Here's how the part is built. I have some questions about the finished solid (model axes, mm). Face numbers are marked on the shaded views. A direction names the side the tool comes from. Round coordinates to 2 decimals unless told otherwise and drop trailing zeros. Write each loop counter-clockwise with the first axis right and the second up, starting at its lowest first coordinate (ties: lowest second). Pieces come first, ordered by that corner, then holes. Notation, with made-up numbers: (62, -31.5) - (100, -31.5) arc R29 ccw to (100, -0.5) - close; hole circle Ø10 at (-23, 33). An arc over 180 degrees is marked (long way). Write item = value, one per line. Start each with the question number.
Item 1: Thinking about a two-plate mould opening in Y: for the marked faces 3, 4, 5 and 6, which applies, pulls with the +Y half, pulls with the -Y half, needs draft (parallel to the pull), parting line crosses it, or undercut?
Item 2: Which directions (+Z, -Z, +X, -X, +Y, -Y) give clear straight access to the entire face, cutting with the end or side of a thin tool? Please do the marked faces 1 and 2.
Item 3: If we section it at B-B (z = 16): Please give me the cut outline in (x, y), and give its area (3 significant figures).
Item 4: If we section it at C-C (x = -2.5): Please give me the cut outline in (y, z), and give its area (3 significant figures).
Item 5: If I drill on line 1 along Z through (x, y) = (-2.5, -1); line 2 along Y through (x, z) = (-5.25, -3); line 3 along Z through (x, y) = (-1, -0.5), over which ranges is the centre line in solid material (lowest first)? Write a range as [from, to].
Item 6: For P1, Ø5, axis at x = -5, y = 9.5, coming from the -Z side; P2, Ø4.5, axis at y = -5.5, z = 10.5, coming from the -X side; P3, Ø2, axis at x = -5, z = -16.5, coming from the -Y side, each with a flat end and sliding along its axis, tell me the tip position at first contact or that it passes through.
Item 7: If we section it at A-A (y = 0): Please give me the cut outline in (x, z).
Item 8: If we section it at D-D (z = 2.5): Give the number of separate pieces and of enclosed holes in the cut face, and give its area (3 significant figures).
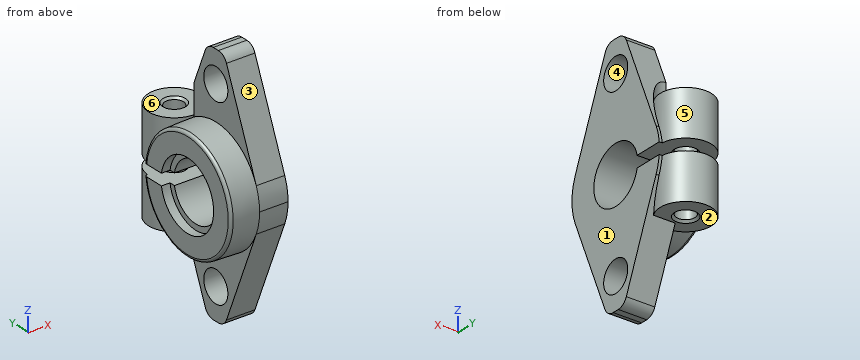
```python
from build123d import *

# Parameters (mm, degrees)
EXTRUDE_1_DEPTH      = 5
EXTRUDE_2_DEPTH      = 9
EXTRUDE_2_DEPTH_BACK = 9
SKETCH_3_R           = 4.5
CUT_EXTRUDE_1_DEPTH  = 9
SKETCH_5_W           = 2
SKETCH_5_H           = 24
CUT_EXTRUDE_2_DEPTH  = 10
SKETCH_9_R           = 2.75
CUT_EXTRUDE_3_DEPTH  = 5
SKETCH_10_R          = 2.75
CUT_EXTRUDE_4_DEPTH  = 5


with BuildPart() as part:
    # 草圖1 → 填料-伸長1 (new body)
    with BuildSketch(Plane(origin=(0, 0, 0), x_dir=(0, 0, -1), z_dir=(1, 0, 0))):
        with BuildLine():
            Line((-21.5, 0.581973136), (-21.5, -0.581973136))
            ThreePointArc((-21.5, -0.581973136), (-21.162939225, -1.693113602), (-20.265366865, -2.429732201))
            Line((-20.265366865, -2.429732201), (-3.826834324, -9.238795325))
            ThreePointArc((-3.826834324, -9.238795325), (-1.95090322, -9.807852804), (0, -10))
            ThreePointArc((0, -10), (1.95090322, -9.807852804), (3.826834324, -9.238795325))
            Line((3.826834324, -9.238795325), (20.265366865, -2.429732201))
            ThreePointArc((20.265366865, -2.429732201), (21.162939225, -1.693113602), (21.5, -0.581973136))
            Line((21.5, -0.581973136), (21.5, 0.581973136))
            ThreePointArc((21.5, 0.581973136), (21.162939225, 1.693113602), (20.265366865, 2.429732201))
            Line((20.265366865, 2.429732201), (3.826834324, 9.238795325))
            ThreePointArc((3.826834324, 9.238795325), (1.95090322, 9.807852804), (0, 10))
            ThreePointArc((0, 10), (-1.95090322, 9.807852804), (-3.826834324, 9.238795325))
            Line((-3.826834324, 9.238795325), (-20.265366865, 2.429732201))
            ThreePointArc((-20.265366865, 2.429732201), (-21.162939225, 1.693113602), (-21.5, 0.581973136))
        make_face()
    extrude(amount=-EXTRUDE_1_DEPTH)

    # 草圖2 → 旋轉1 (revolve)
    with BuildSketch(Plane.XY, mode=Mode.PRIVATE) as revolve_1_sk:
        with BuildLine():
            Line((-10, 0), (-10, 9.334826255))
            ThreePointArc((-10, 9.334826255), (-9.857424619, 9.687712707), (-9.509728944, 9.842516795))
            Line((-9.509728944, 9.842516795), (-5, 10))
            Line((-5, 10), (-5, 0))
            Line((-5, 0), (-10, 0))
        make_face()
    revolve(revolve_1_sk.sketch.rotate(Axis((-5, 0, 0), (-1, 0, 0)), 270), axis=Axis((-5, 0, 0), (-1, 0, 0)))

    # 草圖3 → 填料-伸長2 (add, two sides: drawn at the far end of the back side and taken through both)
    with BuildSketch(Plane.XY.offset(-EXTRUDE_2_DEPTH_BACK)):
        with Locations((-5, 9.5)):
            Circle(SKETCH_3_R)
    extrude(amount=EXTRUDE_2_DEPTH + EXTRUDE_2_DEPTH_BACK)

    # 草圖4 → 除料-伸長1 (cut)
    with BuildSketch(Plane.XY.offset(9)):
        with BuildLine():
            Line((-10, 5), (-5, 5))
            ThreePointArc((-5, 5), (-1.818019485, 12.681980515), (-9.5, 9.5))
            Line((-9.5, 9.5), (-10, 9.5))
            Line((-10, 9.5), (-10, 5))
        make_face()
    extrude(amount=CUT_EXTRUDE_1_DEPTH, mode=Mode.SUBTRACT)

    # 草圖5 → 除料-伸長2 (cut)
    with BuildSketch(Plane(origin=(0, 0, 0), x_dir=(0, 0, -1), z_dir=(1, 0, 0))):
        with Locations((0, 12)):
            Rectangle(SKETCH_5_W, SKETCH_5_H)
    extrude(amount=-CUT_EXTRUDE_2_DEPTH, mode=Mode.SUBTRACT)

    # 草圖6 → 除料-旋轉1 (revolve, cut)
    with BuildSketch(Plane.XY):
        Polygon((-10, 0), (-10, 6), (-8.5, 6), (-8.5, 5), (0, 5), (0, 0), align=None)
    revolve(axis=Axis((0, 0, 0), (-1, 0, 0)), mode=Mode.SUBTRACT)

    # 草圖7 → 除料-旋轉2 (revolve, cut)
    with BuildSketch(Plane(origin=(-5, 0, 0), x_dir=(0, 0, -1), z_dir=(1, 0, 0)), mode=Mode.PRIVATE) as cut_revolve_2_sk:
        Polygon((1, 9.5), (1, 11.5), (1.379, 11.121), (8.621, 11.121), (9.1, 11.6), (13.5, 11.6), (13.5, 9.5), align=None)
    revolve(cut_revolve_2_sk.sketch.rotate(Axis((-5, 9.5, -13.5), (0, 0, 1)), 270), axis=Axis((-5, 9.5, -13.5), (0, 0, 1)), mode=Mode.SUBTRACT)

    # 草圖8 → 除料-旋轉3 (revolve, cut)
    with BuildSketch(Plane(origin=(-5, 0, 0), x_dir=(0, 0, -1), z_dir=(1, 0, 0)), mode=Mode.PRIVATE) as cut_revolve_3_sk:
        Polygon((-9, 9.5), (-9, 11.5), (-8.621, 11.121), (-1.379, 11.121), (-1, 11.5), (-1, 9.5), align=None)
    revolve(cut_revolve_3_sk.sketch.rotate(Axis((-5, 9.5, 1), (0, 0, 1)), 270), axis=Axis((-5, 9.5, 1), (0, 0, 1)), mode=Mode.SUBTRACT)

    # 草圖9 → 除料-伸長3 (cut)
    with BuildSketch(Plane(origin=(0, 0, 0), x_dir=(0, 0, -1), z_dir=(1, 0, 0))):
        with Locations((16, 0)):
            Circle(SKETCH_9_R)
    extrude(amount=-CUT_EXTRUDE_3_DEPTH, mode=Mode.SUBTRACT)

    # 草圖10 → 除料-伸長4 (cut)
    with BuildSketch(Plane(origin=(0, 0, 0), x_dir=(0, 0, -1), z_dir=(1, 0, 0))):
        with Locations((-16, 0)):
            Circle(SKETCH_10_R)
    extrude(amount=-CUT_EXTRUDE_4_DEPTH, mode=Mode.SUBTRACT)


solid = part.part
```
Reply:
q1.face_3 = pulls with the -Y half
q1.face_4 = undercut
q1.face_5 = undercut
q1.face_6 = needs draft
q2.face_1 = +Z, -Z, +X, +Y, -Y
q2.face_2 = -Z, -X, +Y
q3.outline = (-5, -4.2) - (0, -4.2) - (0, -2.75) - (-5, -2.75) - close; (-5, 2.75) - (0, 2.75) - (0, 4.2) - (-5, 4.2) - close
q3.area = 14.5 mm2
q4.outline = (-9.24, -3.83) - (-2.43, -20.27) arc R2 ccw to (-0.58, -21.5) - (0.58, -21.5) arc R2 ccw to (2.43, -20.27) - (7.1, -9) - (13.24, -9) - (13.24, -1) - (4.9, -1) arc R5 cw (long way) to (4.9, 1) - (13.24, 1) - (13.24, 9) - (5.76, 9) - (5.76, 12.23) - (2.43, 20.27) arc R2 ccw to (0.58, 21.5) - (-0.58, 21.5) arc R2 ccw to (-2.43, 20.27) - (-9.24, 3.83) arc R10 ccw to start; hole circle Ø5.5 at (0, -16); hole circle Ø5.5 at (0, 16)
q4.area = 477 mm2
q5.line_1 = [-21.46, -18.56], [-13.44, -4.9], [4.9, 13.44], [18.56, 21.46]
q5.line_2 = [-9.53, -4], [4, 7.9], [11.1, 13.99]
q5.line_3 = [-21.5, -18.7], [-13.3, -4.97], [4.97, 13.3], [18.7, 21.5]
q6.P1 = -9.23
q6.P2 = -9.92
q6.P3 = -4.4
q7.outline = (-10, -9.33) arc R0.51 ccw to (-9.51, -9.84) - (-5, -10) - (-5, -13.25) - (0, -13.25) - (0, -5) - (-8.5, -5) - (-8.5, -6) - (-10, -6) - close; (-10, 6) - (-8.5, 6) - (-8.5, 5) - (0, 5) - (0, 13.25) - (-5, 13.25) - (-5, 10) - (-9.51, 9.84) arc R0.51 ccw to (-10, 9.33) - close; (-5, -21.5) - (0, -21.5) - (0, -18.75) - (-5, -18.75) - close; (-5, 18.75) - (0, 18.75) - (0, 21.5) - (-5, 21.5) - close
q8.separate_pieces = 2
q8.enclosed_holes = 1
q8.area = 125 mm2
